Source: CAD feature listing. Evaluate the final solid. Frame: model axes, mm. A direction names the side the tool comes from. Give positions to 0.01 mm unless a question says otherwise; leave off trailing zeros. Order: outer loops, then holes, each group sorted by start corner. A loop starts at its lowest first (then second) coordinate and runs counter-clockwise, first axis right, second up. Notation, with made-up numbers: M 10.5,31.5 L 60.5,31.5 A21 ccw 60.5,49.5 Z; hole C 36,74 d1. An arc over 180 degrees is marked long. Use CSV: the item, a comma, the result in double quotes. Start each with the question number.
Item 1: Section query A-A on z = -7.25. Return loops of the section in (x, y), and give its area (3 significant figures).
Item 2: First-contact query: pin 1 (1.1 mm diameter, centred on y = 0, z = 1.5, fed in from -X); pin 2 (1.1 mm diameter, centred on y = 0, z = 1, fed in from +X). Flat tips, straight axial feed; report the tip coordinate or a pass-through.
Item 3: Pull-direction query (X, two-part tool) for faces 1 (the face through (-0.6, 0.01, 0.38)), 2 (the face through (0, -2, 0)), 3 (the face through (-0.295, 0.528, 0.382)), 4 (the face through (1.43, -0.45, -5.82)); classes: +X half, -X half, draft (parallel to the pull), parting line (faces both ways), or undercut.
Item 4: Ray query, probe 1 along Y at (x, z) = (0, -1.75); probe 2 along Y at (x, z) = (1.35, -10); probe 3 along X at (y, z) = (1.25, -11.25). Return the intervals inside material, ascending. Write a range as from..to.
Item 5: Access query for faces 5 (the face through (-0.31, -0.52, 0.38)), 6 (the face through (0, 0, -12)). Directions: +Z, -Z, +X, -X, +Y, -Y. A direction counts if a zero-diameter tool reaches every point of the face in a straight line with its end or side. Return the directions, or none.
from build123d import *
from OCP.BRepFilletAPI import BRepFilletAPI_MakeChamfer

# Parameters (mm, degrees)
SKETCH_1_R          = 2.85
EXTRUDE_1_DEPTH     = 1.65
FILLET_1_R          = 1.65
SKETCH_3_R          = 1.5
EXTRUDE_3_DEPTH     = 12
CUT_EXTRUDE_1_DEPTH = 1.616368876
CHAMFER_2_SIZE      = 0.3
CHAMFER_3_SIZE      = 0.576368876
CHAMFER_3_SIZE2     = 0.998300177
FILLET_2_R          = 0.1


with BuildPart() as part:
    # 草图1 → 凸台-拉伸1 (new body)
    with BuildSketch(Plane.XY):
        Circle(SKETCH_1_R)
    extrude(amount=EXTRUDE_1_DEPTH)

    # 圆角1
    fillet_1_edges = [part.edges().sort_by_distance(p)[0] for p in [
        (-2.85, 0, 1.65),
    ]]
    fillet(fillet_1_edges, radius=FILLET_1_R - 0.0001)  # a hair under: the kernel refuses the full size

    # 草图3 → 凸台-拉伸3 (add)
    with BuildSketch(Plane(origin=(0, 0, 0), x_dir=(-1, 0, 0), z_dir=(0, 0, -1))):
        with Locations(Location((0, 0, 0), (0, 0, 180))):
            Circle(SKETCH_3_R)
    extrude(amount=EXTRUDE_3_DEPTH)

    # 草图4 → 切除-拉伸1 (cut)
    with BuildSketch(Plane.XY.offset(1.65)):
        Polygon((1, 0.577350269), (0, 1.154700538), (-1, 0.577350269), (-1, -0.577350269), (0, -1.154700538), (1, -0.577350269), align=None)
    extrude(amount=-CUT_EXTRUDE_1_DEPTH, mode=Mode.SUBTRACT)

    # 倒角2
    chamfer_2_edges = [part.edges().sort_by_distance(p)[0] for p in [
        (-1.5, 0, -12),
    ]]
    chamfer(chamfer_2_edges, length=CHAMFER_2_SIZE)

    # 倒角3: one chamfer whose edges measure the first distance from different faces: ONE call of the kernel's chamfer builder (chamfer() names one face for all edges)
    chamfer_3_edges_1 = [part.edges().sort_by_distance(p)[0] for p in [
        (1, 0, 0.033631124),
    ]]
    chamfer_3_side_1 = [part.faces().sort_by_distance(p)[0] for p in [
        (1, 0, 0.841815562),
    ]]
    chamfer_3_edges_2 = [part.edges().sort_by_distance(p)[0] for p in [
        (0.5, -0.866025404, 0.033631124),
    ]]
    chamfer_3_side_2 = [part.faces().sort_by_distance(p)[0] for p in [
        (0.5, -0.866025404, 0.841815562),
    ]]
    chamfer_3_edges_3 = [part.edges().sort_by_distance(p)[0] for p in [
        (-0.5, -0.866025404, 0.033631124),
    ]]
    chamfer_3_side_3 = [part.faces().sort_by_distance(p)[0] for p in [
        (-0.5, -0.866025404, 0.841815562),
    ]]
    chamfer_3_edges_4 = [part.edges().sort_by_distance(p)[0] for p in [
        (-1, 0, 0.033631124),
    ]]
    chamfer_3_side_4 = [part.faces().sort_by_distance(p)[0] for p in [
        (-1, 0, 0.841815562),
    ]]
    chamfer_3_edges_5 = [part.edges().sort_by_distance(p)[0] for p in [
        (-0.5, 0.866025404, 0.033631124),
    ]]
    chamfer_3_side_5 = [part.faces().sort_by_distance(p)[0] for p in [
        (-0.5, 0.866025404, 0.841815562),
    ]]
    chamfer_3_edges_6 = [part.edges().sort_by_distance(p)[0] for p in [
        (0.5, 0.866025404, 0.033631124),
    ]]
    chamfer_3_side_6 = [part.faces().sort_by_distance(p)[0] for p in [
        (0.5, 0.866025404, 0.841815562),
    ]]
    chamfer_3 = BRepFilletAPI_MakeChamfer(part.part.solid().wrapped)
    for e in chamfer_3_edges_1:
        chamfer_3.Add(CHAMFER_3_SIZE, CHAMFER_3_SIZE2, e.wrapped, chamfer_3_side_1[0].wrapped)  # the first distance lies on this face
    for e in chamfer_3_edges_2:
        chamfer_3.Add(CHAMFER_3_SIZE, CHAMFER_3_SIZE2, e.wrapped, chamfer_3_side_2[0].wrapped)  # the first distance lies on this face
    for e in chamfer_3_edges_3:
        chamfer_3.Add(CHAMFER_3_SIZE, CHAMFER_3_SIZE2, e.wrapped, chamfer_3_side_3[0].wrapped)  # the first distance lies on this face
    for e in chamfer_3_edges_4:
        chamfer_3.Add(CHAMFER_3_SIZE, CHAMFER_3_SIZE2, e.wrapped, chamfer_3_side_4[0].wrapped)  # the first distance lies on this face
    for e in chamfer_3_edges_5:
        chamfer_3.Add(CHAMFER_3_SIZE, CHAMFER_3_SIZE2, e.wrapped, chamfer_3_side_5[0].wrapped)  # the first distance lies on this face
    for e in chamfer_3_edges_6:
        chamfer_3.Add(CHAMFER_3_SIZE, CHAMFER_3_SIZE2, e.wrapped, chamfer_3_side_6[0].wrapped)  # the first distance lies on this face
    add(Compound.cast(chamfer_3.Shape()), mode=Mode.REPLACE)

    # 圆角2
    fillet_2_edges = [part.edges().sort_by_distance(p)[0] for p in [
        (-1.5, 0, 0),
    ]]
    fillet(fillet_2_edges, radius=FILLET_2_R)


solid = part.part
Verdict:
1,outline,"C 0,0 d3"
1,area,"7.07 mm2"
2,pin 1,"x = -2.55"
2,pin 2,"x = 2.79"
3,face 1,"undercut"
3,face 2,"draft"
3,face 3,"undercut"
3,face 4,"parting line"
4,probe 1,"-1.5..1.5"
4,probe 2,"-0.65..0.65"
4,probe 3,"-0.83..0.83"
5,face 5,"+Z"
5,face 6,"-Z, +X, -X, +Y, -Y"
